Read the model definition and answer for the solid it produces. Units are mm, in the model's axes. A direction names the side the tool comes from. Round coordinates to 2 decimals unless told otherwise and drop trailing zeros. Write each loop counter-clockwise with the first axis right and the second up, starting at its lowest first coordinate (ties: lowest second). Pieces come first, ordered by that corner, then holes. Notation, with made-up numbers: (71, 48) -> (97, 48) arc R22 ccw to (97, 64) -> close; hole circle Ø9 at (-31.75, 18). An arc over 180 degrees is marked (long way). Return JSON: item names as keys, results as strings.
from build123d import *

# Parameters (mm, degrees)
F0_R     = 6.5
F1_DEPTH = 125
F2_R     = 2


with BuildPart() as f1:
    # F0 (on Front) → F1 (new body)
    with BuildSketch(Plane.XZ):
        Polygon((-16, 22.055958), (-16, -17.944042), (0, -17.944042), (0, -9.944042), (40, -9.944042), (40, -17.944042), (56, -17.944042), (56, 22.055958), (48, 22.055958), (48, 30.055958), (56, 30.055958), (56, 70.055958), (48, 70.055958), (26, 40.59356), (26, 32.59356), (20, 32.59356), (14, 32.59356), (14, 40.59356), (-8, 70.055958), (-16, 70.055958), (-16, 30.055958), (-8, 30.055958), (-8, 22.055958), align=None)
        with Locations((20, 13.635462)):
            Circle(F0_R, mode=Mode.SUBTRACT)
    extrude(amount=F1_DEPTH)

    # F2
    f2_edges = [f1.edges().sort_by_distance(p)[0] for p in [
        (-16, -125, 50.055958),
        (-12, -125, 70.055958),
        (3, -125, 55.324759),
        (-12, -125, 30.055958),
        (-8, -125, 26.055958),
        (-12, -125, 22.055958),
        (-16, -125, 2.055958),
        (-8, -125, -17.944042),
        (0, -125, -13.944042),
        (20, -125, -9.944042),
        (40, -125, -13.944042),
        (48, -125, -17.944042),
        (56, -125, 2.055958),
        (52, -125, 22.055958),
        (48, -125, 26.055958),
        (52, -125, 30.055958),
        (56, -125, 50.055958),
        (52, -125, 70.055958),
        (37, -125, 55.324759),
        (26, -125, 36.59356),
        (20, -125, 32.59356),
        (14, -125, 36.59356),
        (13.5, -125, 13.635462),
        (-16, 0, 50.055958),
        (-12, 0, 30.055958),
        (-8, 0, 26.055958),
        (-12, 0, 22.055958),
        (-16, 0, 2.055958),
        (-8, 0, -17.944042),
        (0, 0, -13.944042),
        (20, 0, -9.944042),
        (40, 0, -13.944042),
        (48, 0, -17.944042),
        (56, 0, 2.055958),
        (52, 0, 22.055958),
        (48, 0, 26.055958),
        (52, 0, 30.055958),
        (56, 0, 50.055958),
        (52, 0, 70.055958),
        (37, 0, 55.324759),
        (26, 0, 36.59356),
        (20, 0, 32.59356),
        (14, 0, 36.59356),
        (3, 0, 55.324759),
        (-12, 0, 70.055958),
        (13.5, 0, 13.635462),
    ]]
    fillet(f2_edges, radius=F2_R)


solid = f1.part
Item 1: A tool of negligible diameter and unlimited length cuts with its end or side. For faces 5 (the flat face through (0, -62, -14)), 6 (the flat face through (14, -62, 37)), 7 (the flat face through (20, 0, 27)), 8 (the cylindrical face through (37.303, -0.601, 54.777)), 9 (the flat face through (48, -62, 26)), from which of +Z, -Z, +X, -X, +Y, -Y can it reach the whole face along a straight path? Write none if from no direction.
Worked answers:
{"face 5": "-Z, +Y, -Y", "face 6": "+Z, +Y, -Y", "face 7": "+Z, -Z, +X, -X, +Y", "face 8": "+Z, +Y", "face 9": "+X, +Y, -Y"}
Item 2: For a pull along X with two mould halves and no side action, classify faces 1 (the flat face through (52, -62, 22.056)), 2 (the flat face through (26, -62, 37)), 3 (the flat face through (-16, -62, 2)), 4 (the cylindrical face through (2.39, -124.4, 55.19)) as released by +X, released by -X, zero draft, split by the parting line, or undercut.
Worked answers:
{"face 1": "zero draft", "face 2": "undercut", "face 3": "released by -X", "face 4": "undercut"}
Item 3: Flat-ended cylindrical pins translate along their axes: pin 1 (1 mm diameter, centred on y = -67, z = 29.5, fed in from +X); pin 2 (5 mm diameter, centred on x = 39, y = -94.5, fed in from +Z); pin 3 (4 mm diameter, centred on y = -64, z = 27.5, fed in from -X); pin 4 (8 mm diameter, centred on x = 21, z = 21.5, fed in from -Y). Find the tip coordinate at first contact, or state that the pin passes through.
Worked answers:
{"pin 1": "stops at x = 48", "pin 2": "stops at z = 61.35", "pin 3": "stops at x = -8", "pin 4": "stops at y = -125"}
Item 4: Section A-A (x = 20) is taken. Give the vertices of the cut face in (y, z), then the cut area to 3 significant figures.
Worked answers:
{"outline": "(-125, -7.94) arc R2 ccw to (-123, -9.94) -> (-2, -9.94) arc R2 ccw to (0, -7.94) -> (0, 5.14) arc R2 ccw to (-2, 7.14) -> (-123, 7.14) arc R2 ccw to (-125, 5.14) -> close; (-125, 22.14) arc R2 ccw to (-123, 20.14) -> (-2, 20.14) arc R2 ccw to (0, 22.14) -> (0, 30.59) arc R2 ccw to (-2, 32.59) -> (-123, 32.59) arc R2 ccw to (-125, 30.59) -> close", "area": "3,690 mm2"}
Item 5: Straight lines are drawn through the part: L1, parallel to Z at x = 20, y = -30.5; L2, parallel to X at y = -91.5, z = 34; L3, parallel to Z at x = 19.5, y = -53.5. For each, find the intervals that lie inside material, in ascending order. Write a range as [from, to].
Worked answers:
{"L1": "z = [-9.94, 7.14], [20.14, 32.59]", "L2": "x = [-16, 14], [26, 56]", "L3": "z = [-9.94, 7.15], [20.12, 32.59]"}
Item 6: Section B-B (y = -56.5) is taken. Give the vertices of the cut face in (x, z).
Worked answers:
{"outline": "(-16, -17.94) -> (0, -17.94) -> (0, -9.94) -> (40, -9.94) -> (40, -17.94) -> (56, -17.94) -> (56, 22.06) -> (48, 22.06) -> (48, 30.06) -> (56, 30.06) -> (56, 70.06) -> (48, 70.06) -> (26, 40.59) -> (26, 32.59) -> (14, 32.59) -> (14, 40.59) -> (-8, 70.06) -> (-16, 70.06) -> (-16, 30.06) -> (-8, 30.06) -> (-8, 22.06) -> (-16, 22.06) -> close; hole circle Ø13 at (20, 13.64)"}
